Read the model definition and answer for the solid it produces. Units are mm, in the model's axes. A direction names the side the tool comes from. Round coordinates to 2 decimals unless told otherwise and drop trailing zeros. Order: outer loops, then holes, each group sorted by start corner. A loop starts at its lowest first (then second) coordinate and runs counter-clockwise, first axis right, second up. Notation, with made-up numbers: (43.25, 29.25) -> (99.25, 29.25) arc R19 cw to (99.25, 46.25) -> close; hole circle Ø9 at (43.25, 72.5). An arc over 180 degrees is marked (long way). Use a Markdown table: item, result. Add a question column.
1. Given pin 1 (1 mm diameter, centred on x = -106, y = -410.5, fed in from +Z); pin 2 (3 mm diameter, centred on x = -106.5, z = 63, fed in from -Y); pin 3 (1.1 mm diameter, centred on x = -106, y = -221.5, fed in from -Z), each flat-ended and moving along its own axis, determine where each tip first touches the part or whether it passes through.
2. Section B-B, the plane x = -108.35 is taken. Give the number of separate pieces and of enclosed holes in the cut face, then the cut area to 3 significant figures.
3. The mould has two halves that part along Z. Classify faces 1 (the face through (-107, -210, 59)), 2 (the face through (-106.958, -466.292, 12.803)), 3 (the face through (-107, -424.604, 62)): +Z half, -Z half, draft (parallel to the pull), parting line (faces both ways), or undercut.
4. For faces 4 (the face through (-107, -353.054, 3)), 5 (the face through (-106.958, -464.694, 40.548)), 6 (the face through (-107, -452.154, 56)), 7 (the face through (-107, -231.604, 12)), determine the directions among +Z, -Z, +X, -X, +Y, -Y from which every point of the face is accessible in a straight line to the end or side of a thin tool.
5. Section A-A, the plane y = -297.5 is taken. Give the vertices of the cut face in (x, z).
6. Consider L1, parallel to Y at x = -104.65, z = 60; L2, parallel to Y at x = -105.05, z = 8; L3, parallel to Y at x = -107.25, z = 33.5. Determine where each line is inside the solid, lowest interval first. Write a range as [from, to].
```python
from build123d import *

# Parameters (mm, degrees)
DODANIE_WYCI_GNI_CIE1_DEPTH      = 65
DODANIE_WYCI_GNI_CIE1_DEPTH_BACK = 6.5
SZKIC1_W                         = 6
SZKIC1_H                         = 318
WYTNIJ_WYCI_GNI_CIE1_DEPTH       = 6
SZKIC4_W                         = 6
SZKIC4_H                         = 253
WYTNIJ_WYCI_GNI_CIE2_DEPTH       = 6
WYTNIJ_WYCI_GNI_CIE3_DEPTH       = 6
SZYK_LINIOWY2_COUNT              = 2
SZYK_LINIOWY2_PITCH              = 100
SZYK_LINIOWY2_COL_COUNT          = 2
SZYK_LINIOWY2_COL_PITCH          = 200
SZKIC6_W                         = 6
SZKIC6_H                         = 40
WYTNIJ_WYCI_GNI_CIE4_DEPTH       = 6
SZYK_LINIOWY3_COUNT              = 6
SZYK_LINIOWY3_PITCH              = 60
SZYK_LINIOWY3_COUNT_DIR2         = 2
SZYK_LINIOWY3_PITCH_DIR2         = 250
WYTNIJ_WYCI_GNI_CIE5_DEPTH       = 6
SZYK_LINIOWY4_COUNT              = 2
SZYK_LINIOWY4_PITCH              = 107
SZYK_LINIOWY4_COL_COUNT          = 2
SZYK_LINIOWY4_COL_PITCH          = 227
SZKIC9_R                         = 1.55
WYTNIJ_WYCI_GNI_CIE6_DEPTH       = 6
WYTNIJ_WYCI_GNI_CIE7_DEPTH       = 6
SZKIC13_R                        = 1.55
WYTNIJ_WYCI_GNI_CIE9_DEPTH       = 10


with BuildPart() as part:
    # Szkic1 → Dodanie-wyciągnięcie1 (new, two sides: drawn at the far end of the back side and taken through both)
    with BuildSketch(Plane.XY.offset(-DODANIE_WYCI_GNI_CIE1_DEPTH_BACK)):
        with Locations((-107, -325.603962956)):
            Rectangle(SZKIC1_W, SZKIC1_H)
    extrude(amount=DODANIE_WYCI_GNI_CIE1_DEPTH + DODANIE_WYCI_GNI_CIE1_DEPTH_BACK)

    # Szkic2 → Wytnij-wyciągnięcie1 (cut)
    with BuildSketch(Plane.ZY.offset(110)):
        Polygon((-6.5, -231.603962956), (25.5, -231.603962956), (25.5, -196.603962956), (65, -196.603962956), (65, -166.603962956), (-6.5, -166.603962956), align=None)
    extrude(amount=-WYTNIJ_WYCI_GNI_CIE1_DEPTH, mode=Mode.SUBTRACT)

    # Szkic4 → Wytnij-wyciągnięcie2 (cut)
    with BuildSketch(Plane.ZY.offset(110)):
        with Locations((-3.5, -358.103962956)):
            Rectangle(SZKIC4_W, SZKIC4_H)
    extrude(amount=-WYTNIJ_WYCI_GNI_CIE2_DEPTH, mode=Mode.SUBTRACT)

    # Szkic5 → Wytnij-wyciągnięcie3 (cut)
    with BuildSketch(Plane.ZY.offset(110)):
        Polygon((-0.5, -453.053962956), (-0.5, -456.153962956), (6.5, -456.153962956), (6.5, -457.528962956), (8.5, -457.528962956), (8.5, -456.153962956), (9, -456.153962956), (9, -453.053962956), (8.5, -453.053962956), (8.5, -451.678962956), (6.5, -451.678962956), (6.5, -453.053962956), align=None)
    wytnij_wyci_gni_cie3 = extrude(amount=-WYTNIJ_WYCI_GNI_CIE3_DEPTH, mode=Mode.SUBTRACT)

    # Szyk liniowy2: Wytnij-wyciągnięcie3 ×2
    with Locations(*[(0, i * SZYK_LINIOWY2_PITCH, 0) for i in range(1, SZYK_LINIOWY2_COUNT)]):
        add(wytnij_wyci_gni_cie3, mode=Mode.SUBTRACT)

    # Szyk liniowy2 col: Wytnij-wyciągnięcie3 ×2
    with Locations(*[(0, i * SZYK_LINIOWY2_COL_PITCH, 0) for i in range(1, SZYK_LINIOWY2_COL_COUNT)]):
        add(wytnij_wyci_gni_cie3, mode=Mode.SUBTRACT)

    # Szkic6 → Wytnij-wyciągnięcie4 (cut)
    with BuildSketch(Plane(origin=(-104, 0, 0), x_dir=(0, 0, -1), z_dir=(1, 0, 0))):
        with Locations((-62, -464.603962956)):
            Rectangle(SZKIC6_W, SZKIC6_H)
    wytnij_wyci_gni_cie4 = extrude(amount=-WYTNIJ_WYCI_GNI_CIE4_DEPTH, mode=Mode.SUBTRACT)

    # Szyk liniowy3: Wytnij-wyci_gni_cie4 6 × 2
    with Locations(*[Vector(0, 1, 0) * (i * SZYK_LINIOWY3_PITCH) + Vector(0, 1, 0) * (j * SZYK_LINIOWY3_PITCH_DIR2) for i in range(SZYK_LINIOWY3_COUNT) for j in range(SZYK_LINIOWY3_COUNT_DIR2) if (i, j) != (0, 0)]):
        add(wytnij_wyci_gni_cie4, mode=Mode.SUBTRACT)

    # Szkic7 → Wytnij-wyciągnięcie5 (cut)
    with BuildSketch(Plane(origin=(-104, 0, 0), x_dir=(0, 0, -1), z_dir=(1, 0, 0))):
        Polygon((-59, -449.053962956), (-59, -452.153962956), (-52, -452.153962956), (-52, -453.528962956), (-50, -453.528962956), (-50, -452.153962956), (-49.5, -452.153962956), (-49.5, -449.053962956), (-50, -449.053962956), (-50, -447.678962956), (-52, -447.678962956), (-52, -449.053962956), align=None)
    wytnij_wyci_gni_cie5 = extrude(amount=-WYTNIJ_WYCI_GNI_CIE5_DEPTH, mode=Mode.SUBTRACT)

    # Szyk liniowy4: Wytnij-wyciągnięcie5 ×2
    with Locations(*[(0, i * SZYK_LINIOWY4_PITCH, 0) for i in range(1, SZYK_LINIOWY4_COUNT)]):
        add(wytnij_wyci_gni_cie5, mode=Mode.SUBTRACT)

    # Szyk liniowy4 col: Wytnij-wyciągnięcie5 ×2
    with Locations(*[(0, i * SZYK_LINIOWY4_COL_PITCH, 0) for i in range(1, SZYK_LINIOWY4_COL_COUNT)]):
        add(wytnij_wyci_gni_cie5, mode=Mode.SUBTRACT)

    # Szkic9 → Wytnij-wyciągnięcie6 (cut)
    with BuildSketch(Plane.ZY.offset(110)):
        with Locations(Location((32.500000044, -481.603962956, 0), (0, 0, 270))):
            Circle(SZKIC9_R)
    extrude(amount=-WYTNIJ_WYCI_GNI_CIE6_DEPTH, mode=Mode.SUBTRACT)

    # Szkic11 → Wytnij-wyciągnięcie7 (cut)
    with BuildSketch(Plane(origin=(-104, 0, 0), x_dir=(0, 0, -1), z_dir=(1, 0, 0))):
        Polygon((-19.205244402, -465.162826439), (-6.219752977, -467.452518935), (-7.331101314, -473.755288555), (-20.316592739, -471.465596059), align=None)
        Polygon((-39.98468799, -461.498849891), (-54.165919634, -458.998316132), (-55.277267971, -465.301085752), (-41.096036327, -467.80161951), align=None)
    extrude(amount=-WYTNIJ_WYCI_GNI_CIE7_DEPTH, mode=Mode.SUBTRACT)

    # Szkic13 → Wytnij-wyciągnięcie9 (cut)
    with BuildSketch(Plane.ZY.offset(110)):
        with Locations(Location((50.000000044, -260.153962956, 0), (0, 0, 270))):
            Circle(SZKIC13_R)
        with Locations(Location((50.000000044, -277.053962956, 0), (0, 0, 270))):
            Circle(SZKIC13_R)
    extrude(amount=-WYTNIJ_WYCI_GNI_CIE9_DEPTH, mode=Mode.SUBTRACT)


solid = part.part
```
Verdict:
| question | item | result |
|---|---|---|
| 1 | pin 1 | stops at z = 59 |
| 1 | pin 2 | stops at y = -444.6 |
| 1 | pin 3 | stops at z = 25.5 |
| 2 | separate pieces | 1 |
| 2 | enclosed holes | 5 |
| 2 | area | 16,300 mm2 |
| 3 | face 1 | +Z half |
| 3 | face 2 | undercut |
| 3 | face 3 | draft |
| 4 | face 4 | -Z, +X, -X |
| 4 | face 5 | +X, -X |
| 4 | face 6 | +Z, +X, -X |
| 4 | face 7 | -Z, +X, -X, +Y |
| 5 | outline | (-110, -0.5) -> (-104, -0.5) -> (-104, 59) -> (-110, 59) -> close |
| 6 | L1 | y = [-444.6, -424.6], [-384.6, -364.6], [-324.6, -304.6], [-264.6, -244.6] |
| 6 | L2 | y = [-484.6, -473.64], [-467.14, -457.53], [-451.68, -357.53], [-351.68, -257.53], [-251.68, -231.6] |
| 6 | L3 | y = [-484.6, -482.79], [-480.42, -196.6] |
